from build123d import *

# Parameters (mm, degrees)
SKETCH1_R           = 100
BOSS_EXTRUDE1_DEPTH = 100
SKETCH2_W           = 446.6
SKETCH2_H           = 446.6
BOSS_EXTRUDE2_DEPTH = 50


with BuildPart() as part:
    # Sketch1 → Boss-Extrude1 (new body)
    with BuildSketch(Plane.XY):
        Circle(SKETCH1_R)
    extrude(amount=BOSS_EXTRUDE1_DEPTH)

    # Sketch2 → Boss-Extrude2 (add)
    with BuildSketch(Plane(origin=(0, 0, 0), x_dir=(-1, 0, 0), z_dir=(0, 0, -1))):
        Rectangle(SKETCH2_W, SKETCH2_H)
    extrude(amount=BOSS_EXTRUDE2_DEPTH)


solid = part.part
Read the model definition and answer for the solid it produces. Units are mm, in the model's axes. A direction names the side the tool comes from. Coordinates: 2 decimals unless noted, no trailing zeros. Order: outer loops, then holes, each group sorted by start corner. A loop starts at its lowest first (then second) coordinate and runs counter-clockwise, first axis right, second up. Notation, with made-up numbers: M 58,-37.5 L 83,-37.5 A23 cw 83,-5.5 Z; hole C 69,1 d10. An arc over 180 degrees is marked long. Put each result on its own line as item: value. Start each with the question number.
Item 1: Consider probe 1 along Z at (x, y) = (-147.5, -178); probe 2 along X at (y, z) = (-53.5, 39.5); probe 3 along X at (y, z) = (53, 87). Determine where each line is inside the solid, lowest interval first. Write a range as [from, to].
Item 2: Section D-D, the plane x = -145 is taken. Determine the outline of the cut face in (y, z), plus the area to 3 significant figures.
Item 3: Section C-C, the plane z = 32 is taken. Determine the outline of the cut face in (x, y).
Item 4: Section A-A, the plane x = 0 is taken. Determine the outline of the cut face in (y, z), plus the area to 3 significant figures.
Item 5: For faces 1 (the face through (3, 102, 0)), 2 (the face through (-223.3, -3, -25)), determine the directions among +Z, -Z, +X, -X, +Y, -Y from which every point of the face is accessible in a straight line to the end or side of a thin tool.
Item 6: Given pin 1 Ø4 at (x, y) = (172.5, -107.5) entering from +Z; pin 2 Ø2 at (x, z) = (-70.5, 71) entering from -Y, each flat-ended and moving along its own axis, determine where each tip first touches the part or whether it passes through.
Computed:
1. probe 1: z = [-50, 0]
1. probe 2: x = [-84.49, 84.49]
1. probe 3: x = [-84.8, 84.8]
2. outline: M -223.3,-50 L 223.3,-50 L 223.3,0 L -223.3,0 Z
2. area: 22,300 mm2
3. outline: C 0,0 d200
4. outline: M -223.3,-50 L 223.3,-50 L 223.3,0 L 100,0 L 100,100 L -100,100 L -100,0 L -223.3,0 Z
4. area: 42,300 mm2
5. face 1: +Z
5. face 2: +Z, -Z, -X, +Y, -Y
6. pin 1: stops at z = 0
6. pin 2: stops at y = -71.9
